from build123d import *

# Parameters (mm, degrees)
SKETCH_1_R          = 52
EXTRUDE_1_DEPTH     = 20
CUT_EXTRUDE_START   = -20
SKETCH_2_R          = 52
SKETCH_2_R_2        = 51.5
CUT_EXTRUDE_1_DEPTH = 20
SKETCH_3_R          = 51.5
SKETCH_3_R_2        = 1.75
SKETCH_3_R_3        = 35
EXTRUDE_2_DEPTH     = 3
SKETCH_4_W          = 6.656096692
SKETCH_4_H          = 30.90307428
SKETCH_4_W_2        = 11.077487824
CUT_EXTRUDE_2_DEPTH = 77.377352664
EXTRUDE_START       = -3
SKETCH_6_R          = 1.75
SKETCH_6_R_2        = 1.891027651
EXTRUDE_3_DEPTH     = 3
SKETCH_7_R          = 1.75
CUT_EXTRUDE_3_DEPTH = 3


with BuildPart() as part:
    # 草图1 → 凸台-拉伸1 (new body)
    with BuildSketch(Plane(origin=(0, 0, 0), x_dir=(1, 0, 0), z_dir=(0, 1, 0))):
        with Locations(Location((0, 0, 0), (0, 0, 270))):
            Circle(SKETCH_1_R)
        with BuildLine():
            Line((-46.5, -15.45153714), (-46.5, 15.45153714))
            ThreePointArc((-46.5, 15.45153714), (0, 49), (46.5, 15.45153714))
            Line((46.5, 15.45153714), (46.5, -15.45153714))
            ThreePointArc((46.5, -15.45153714), (0, -49), (-46.5, -15.45153714))
        make_face(mode=Mode.SUBTRACT)
    extrude(amount=EXTRUDE_1_DEPTH)

    # 草图2 → 切除-拉伸1 (cut)
    with BuildSketch(Plane(origin=(0, 20, 0), x_dir=(1, 0, 0), z_dir=(0, 1, 0)).offset(CUT_EXTRUDE_START)):
        Circle(SKETCH_2_R)
        with Locations(Location((0, 0, 0), (0, 0, 270))):
            Circle(SKETCH_2_R_2, mode=Mode.SUBTRACT)
    extrude(amount=CUT_EXTRUDE_1_DEPTH, mode=Mode.SUBTRACT)

    # 草图3 → 凸台-拉伸2 (add)
    with BuildSketch(Plane(origin=(0, 20, 0), x_dir=(1, 0, 0), z_dir=(0, 1, 0))):
        with Locations(Location((0, 0, 0), (0, 0, 270))):
            Circle(SKETCH_3_R)
        with Locations(Location((0, 42.5, 0), (0, 0, 270))):
            Circle(SKETCH_3_R_2, mode=Mode.SUBTRACT)
        with Locations(Location((30.0520382, 30.0520382, 0), (0, 0, 270))):
            Circle(SKETCH_3_R_2, mode=Mode.SUBTRACT)
        with Locations(Location((42.5, 0, 0), (0, 0, 270))):
            Circle(SKETCH_3_R_2, mode=Mode.SUBTRACT)
        with Locations(Location((30.0520382, -30.0520382, 0), (0, 0, 270))):
            Circle(SKETCH_3_R_2, mode=Mode.SUBTRACT)
        with Locations(Location((0, -42.5, 0), (0, 0, 270))):
            Circle(SKETCH_3_R_2, mode=Mode.SUBTRACT)
        with Locations(Location((-30.0520382, -30.0520382, 0), (0, 0, 270))):
            Circle(SKETCH_3_R_2, mode=Mode.SUBTRACT)
        with Locations(Location((-42.5, 0, 0), (0, 0, 270))):
            Circle(SKETCH_3_R_2, mode=Mode.SUBTRACT)
        with Locations(Location((-30.0520382, 30.0520382, 0), (0, 0, 270))):
            Circle(SKETCH_3_R_2, mode=Mode.SUBTRACT)
        with Locations(Location((0, 0, 0), (0, 0, 270))):
            Circle(SKETCH_3_R_3, mode=Mode.SUBTRACT)
    extrude(amount=EXTRUDE_2_DEPTH)

    # 草图4 → 切除-拉伸2 (cut, through all)
    with BuildSketch(Plane.XZ):
        with Locations((-52.828048346, 0)):
            Rectangle(SKETCH_4_W, SKETCH_4_H)
        with Locations((55.038743912, 0)):
            Rectangle(SKETCH_4_W_2, SKETCH_4_H)
    extrude(amount=-CUT_EXTRUDE_2_DEPTH, mode=Mode.SUBTRACT)

    # 草图6 → 凸台-拉伸3 (add)
    with BuildSketch(Plane(origin=(0, 23, 0), x_dir=(1, 0, 0), z_dir=(0, 1, 0)).offset(EXTRUDE_START)):
        with Locations((-30.0520382, 30.0520382)):
            Circle(SKETCH_6_R)
        with Locations((0, 42.5)):
            Circle(SKETCH_6_R)
        with Locations((30.0520382, 30.0520382)):
            Circle(SKETCH_6_R)
        with Locations((30.0520382, -30.0520382)):
            Circle(SKETCH_6_R_2)
        with Locations((0, -42.5)):
            Circle(SKETCH_6_R)
        with Locations((-30.0520382, -30.0520382)):
            Circle(SKETCH_6_R)
    extrude(amount=EXTRUDE_3_DEPTH)

    # 草图7 → 切除-拉伸3 (cut)
    with BuildSketch(Plane(origin=(0, 23, 0), x_dir=(1, 0, 0), z_dir=(0, 1, 0))):
        with Locations(Location((0, 44.5, 0), (0, 0, 270))):
            Circle(SKETCH_7_R)
        with Locations(Location((31.466251763, 31.466251763, 0), (0, 0, 270))):
            Circle(SKETCH_7_R)
        with Locations(Location((31.466251763, -31.466251763, 0), (0, 0, 270))):
            Circle(SKETCH_7_R)
        with Locations(Location((0, -44.5, 0), (0, 0, 270))):
            Circle(SKETCH_7_R)
        with Locations(Location((-31.466251763, -31.466251763, 0), (0, 0, 270))):
            Circle(SKETCH_7_R)
        with Locations(Location((-31.466251763, 31.466251763, 0), (0, 0, 270))):
            Circle(SKETCH_7_R)
    extrude(amount=-CUT_EXTRUDE_3_DEPTH, mode=Mode.SUBTRACT)


solid = part.part
Work out the finished part from the listing and answer in its coordinate system (mm). A direction names the side the tool comes from. Give positions to 0.01 mm unless a question says otherwise; leave off trailing zeros. Loops run counter-clockwise (first coordinate to the right, second up) from the corner with the lowest first, then second, coordinate; pieces in that order, holes last. Notation, with made-up numbers: (3.25, -23) -> (60.25, -23) arc R13 ccw to (60.25, -18) -> close; hole circle Ø7 at (77, 9). An arc over 180 degrees is marked (long way). Use a Markdown table: item, result. Add a question column.
1. Section D-D on x = -13 is taken. Determine the outline of the cut face in (y, z).
2. Determine the mould class of faces 1 (the cylindrical face through (0.93, 11.34, -51.49)), 2 (the cylindrical face through (-0.93, 11.34, 51.49)), 3 (the cylindrical face through (-0.67, 21.521, -42.883)), 4 (the cylindrical face through (0.857, 9.86, 48.992)) for opening direction Z: released by +Z, released by -Z, zero draft, split by the parting line, or undercut.
3. Section B-B on x = 0 is taken. Determine the outline of the cut face in (y, z).
4. For faces 5 (the cylindrical face through (-31.389, 21.521, -33.215)), 6 (the flat face through (-46.5, 10, 0)), determine the directions among +Z, -Z, +X, -X, +Y, -Y from which every point of the face is accessible in a straight line to the end or side of a thin tool.
5. Section A-A on z = 0 is taken. Determine the outline of the cut face in (x, y), and give its area (3 significant figures).
6. Find the intervals of material crossed by probe 1 along X at (y, z) = (7.5, 9); probe 2 along Y at (x, z) = (41.5, 24.5); probe 3 along Z at (x, y) = (12, 9.25), in increasing order.
7. Section C-C on y = 5 is taken. Determine the outline of the cut face in (x, z).
8. Flat-ended cylindrical pins translate along their axes: pin 1 Ø3 at (x, z) = (-31.47, -31.47) entering from -Y; pin 2 Ø4.5 at (x, z) = (0, 44.5) entering from -Y; pin 3 Ø6 at (x, y) = (-12.5, 9) entering from +Z; pin 4 Ø3 at (x, y) = (-8, 20) entering from -Z. Find the tip coordinate at first contact, or state that the pin passes through.
Results below:
| question | item | result |
|---|---|---|
| 1 | outline | (0, -49.83) -> (23, -49.83) -> (23, -32.5) -> (20, -32.5) -> (20, -47.24) -> (0, -47.24) -> close; (0, 47.24) -> (20, 47.24) -> (20, 32.5) -> (23, 32.5) -> (23, 49.83) -> (0, 49.83) -> close |
| 2 | face 1 | released by -Z |
| 2 | face 2 | released by +Z |
| 2 | face 3 | undercut |
| 2 | face 4 | undercut |
| 3 | outline | (0, -51.5) -> (23, -51.5) -> (23, -46.25) -> (20, -46.25) -> (20, -49) -> (0, -49) -> close; (0, 49) -> (20, 49) -> (20, 46.25) -> (23, 46.25) -> (23, 51.5) -> (0, 51.5) -> close; (20, -42.75) -> (23, -42.75) -> (23, -35) -> (20, -35) -> close; (20, 35) -> (23, 35) -> (23, 42.75) -> (20, 42.75) -> close |
| 4 | face 5 | +Y, -Y |
| 4 | face 6 | -Y |
| 5 | outline | (-49.5, 0) -> (-46.5, 0) -> (-46.5, 20) -> (-44.25, 20) -> (-44.25, 23) -> (-49.5, 23) -> close; (-40.75, 20) -> (-35, 20) -> (-35, 23) -> (-40.75, 23) -> close; (35, 20) -> (40.75, 20) -> (40.75, 23) -> (35, 23) -> close; (44.25, 20) -> (46.5, 20) -> (46.5, 0) -> (49.5, 0) -> (49.5, 23) -> (44.25, 23) -> close |
| 5 | area | 186 mm^2 |
| 6 | probe 1 | x = -49.5 to -46.5, 46.5 to 49.5 |
| 6 | probe 2 | y = 20 to 23 |
| 6 | probe 3 | z = -50.08 to -47.51, 47.51 to 50.08 |
| 7 | outline | (-49.5, -14.21) arc R51.5 ccw to (49.5, -14.21) -> (49.5, 14.21) arc R51.5 ccw to (-49.5, 14.21) -> close; hole (-46.5, -15.45) arc R49 ccw to (46.5, -15.45) -> (46.5, 15.45) arc R49 ccw to (-46.5, 15.45) -> close |
| 8 | pin 1 | passes through |
| 8 | pin 2 | stops at y = 20 |
| 8 | pin 3 | stops at z = 50.62 |
| 8 | pin 4 | stops at z = -51.09 |
